```python
from build123d import *

# Parameters (mm, degrees)
F0_R     = 14
F1_DEPTH = 7


with BuildPart() as f1:
    # F0 (on Top) → F1 (new body)
    with BuildSketch(Plane.XY):
        Circle(F0_R)
        with BuildLine():
            Line((-8.75, 6.573926), (-5.25, 6.573926))
            ThreePointArc((-5.25, 6.573926), (-4.18934, 6.134586), (-3.75, 5.073926))
            Line((-3.75, 5.073926), (-3.75, -5.073926))
            ThreePointArc((-3.75, -5.073926), (-4.18934, -6.134586), (-5.25, -6.573926))
            Line((-5.25, -6.573926), (-8.75, -6.573926))
            ThreePointArc((-8.75, -6.573926), (-9.81066, -6.134586), (-10.25, -5.073926))
            Line((-10.25, -5.073926), (-10.25, 5.073926))
            ThreePointArc((-10.25, 5.073926), (-9.81066, 6.134586), (-8.75, 6.573926))
        make_face(mode=Mode.SUBTRACT)
        with BuildLine():
            Line((10.25, 5.073926), (10.25, -5.073926))
            ThreePointArc((10.25, -5.073926), (9.81066, -6.134586), (8.75, -6.573926))
            Line((8.75, -6.573926), (5.25, -6.573926))
            ThreePointArc((5.25, -6.573926), (4.18934, -6.134586), (3.75, -5.073926))
            Line((3.75, -5.073926), (3.75, 5.073926))
            ThreePointArc((3.75, 5.073926), (4.18934, 6.134586), (5.25, 6.573926))
            Line((5.25, 6.573926), (8.75, 6.573926))
            ThreePointArc((8.75, 6.573926), (9.81066, 6.134586), (10.25, 5.073926))
        make_face(mode=Mode.SUBTRACT)
    extrude(amount=F1_DEPTH)


solid = f1.part
```
Could you check a few things on this model? Use its own coordinates, in mm. A direction names the side the tool comes from. Coordinates: 2 decimals unless noted, no trailing zeros. Order: outer loops, then holes, each group sorted by start corner. A loop starts at its lowest first (then second) coordinate and runs counter-clockwise, first axis right, second up. Notation, with made-up numbers: M 3,31 L 12,31 A23 cw 12,50 Z; hole C 32.25,88 d1. An arc over 180 degrees is marked long. Use one line per item in the form item = value. Start each with the question number.
1. Suppose I cut it at A-A on y = 0. Write out the boundary of the cut face in (x, z), then the cut area to 3 significant figures.
2. Suppose I cut it at D-D on y = -4. Write out the boundary of the cut face in (x, z), then the cut area to 3 significant figures.
3. On a 3-axis mill with a long thin cutter (end or side, diameter ignored), from which of +Z, -Z, +X, -X, +Y, -Y can I reach the whole of each face in a straight line? I mean faces 5 (the flat face through (0, 0, 7)), 6 (the cylindrical face through (4.201, -6.146, 3.451)). Say none if no direction works.
4. Please list where these lines run through material, in increasing order: line 1 (X direction, y = -1.5, z = 0.5); line 2 (X direction, y = -0.75, z = 1.25); line 3 (Y direction, x = 5, z = 6.5).
5. For pin 1 (4 mm diameter, centred on x = -8.5, z = 3.5, fed in from +Y); pin 2 (4 mm diameter, centred on x = 6.5, z = 5, fed in from +Y); pin 3 (3.5 mm diameter, centred on y = 2, z = 2, fed in from -X), each with a flat end and sliding along its axis, tell me the tip position at first contact or that it passes through.
6. Suppose I cut it at B-B on z = 5.5. Write out the boundary of the cut face in (x, y), then the cut area to 3 significant figures.
7. Suppose I cut it at C-C on x = -7.5. Write out the boundary of the cut face in (y, z).
8. We'd pull the mould along Y, two halves only. Please class faces 1 (the flat face through (0, 0, 0)), 2 (the flat face through (10.25, 0, 3)), 3 (the cylindrical face through (-4.178, -6.123, 3.451)), 4 (the cylindrical face through (12.932, -5.362, 3.451)): +Y half, -Y half, draft (parallel to the pull), parting line (faces both ways), or undercut.
Geometry says:
q1.outline = M -14,0 L -10.25,0 L -10.25,7 L -14,7 Z; M -3.75,0 L 3.75,0 L 3.75,7 L -3.75,7 Z; M 10.25,0 L 14,0 L 14,7 L 10.25,7 Z
q1.area = 105 mm^2
q2.outline = M -13.42,0 L -10.25,0 L -10.25,7 L -13.42,7 Z; M -3.75,0 L 3.75,0 L 3.75,7 L -3.75,7 Z; M 10.25,0 L 13.42,0 L 13.42,7 L 10.25,7 Z
q2.area = 96.8 mm^2
q3.face_5 = +Z, +X, -X, +Y, -Y
q3.face_6 = +Z, -Z
q4.line_1 = -13.92 to -10.25, -3.75 to 3.75, 10.25 to 13.92
q4.line_2 = -13.98 to -10.25, -3.75 to 3.75, 10.25 to 13.98
q4.line_3 = -13.08 to -6.55, 6.55 to 13.08
q5.pin_1 = 12.4
q5.pin_2 = 13.26
q5.pin_3 = -14
q6.outline = C 0,0 d28; hole M -10.25,-5.07 A1.5 ccw -8.75,-6.57 L -5.25,-6.57 A1.5 ccw -3.75,-5.07 L -3.75,5.07 A1.5 ccw -5.25,6.57 L -8.75,6.57 A1.5 ccw -10.25,5.07 Z; hole M 3.75,-5.07 A1.5 ccw 5.25,-6.57 L 8.75,-6.57 A1.5 ccw 10.25,-5.07 L 10.25,5.07 A1.5 ccw 8.75,6.57 L 5.25,6.57 A1.5 ccw 3.75,5.07 Z
q6.area = 449 mm^2
q7.outline = M -11.82,0 L -6.57,0 L -6.57,7 L -11.82,7 Z; M 6.57,0 L 11.82,0 L 11.82,7 L 6.57,7 Z
q8.face_1 = draft
q8.face_2 = undercut
q8.face_3 = undercut
q8.face_4 = parting line
